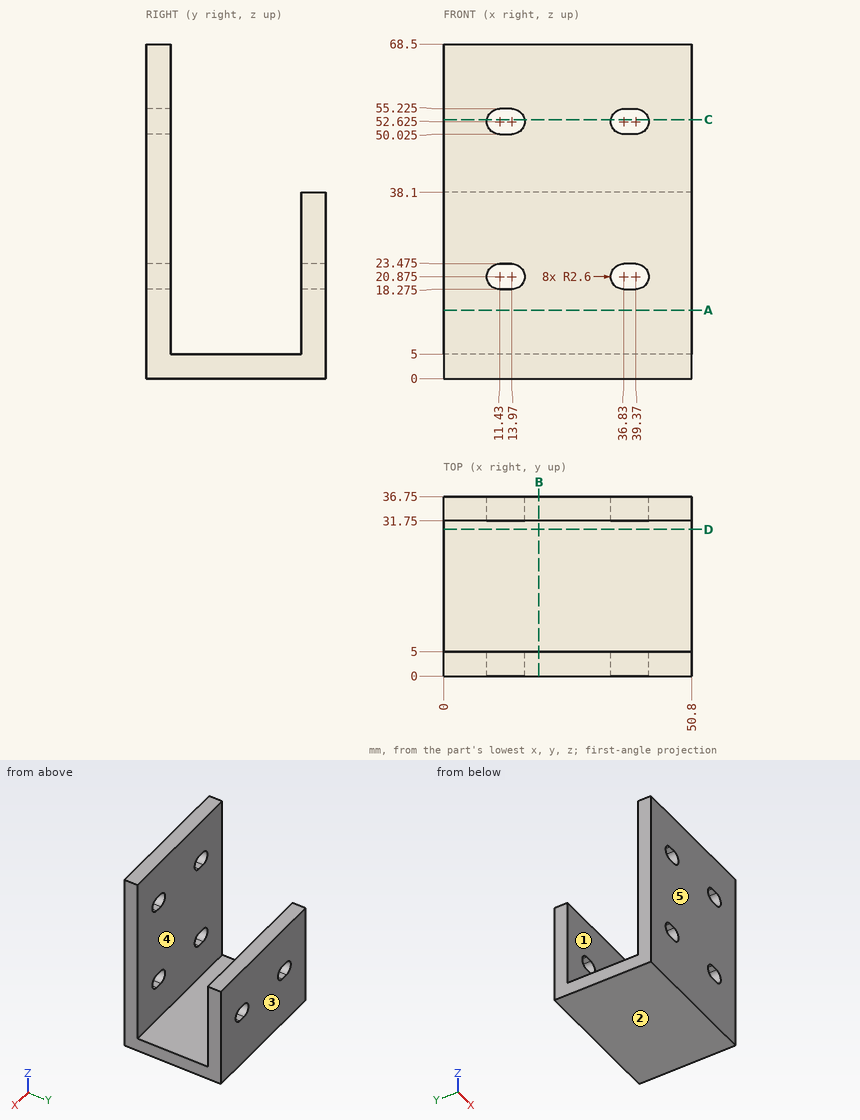
Check sheet for the drawn part. Datum: minimum x, y, z corner. Units: mm. A direction names the side the tool comes from. Round coordinates to 2 decimals unless told otherwise and drop trailing zeros. Loops run counter-clockwise (first coordinate to the right, second up) from the corner with the lowest first, then second, coordinate; pieces in that order, holes last.
Item 1: Mould release check, pull along Y, two halves, no side actions. Record for the marked faces 3, 4 and 5: pulls with the +Y half, pulls with the -Y half, needs draft (parallel to the pull), parting line crosses it, or undercut.
Item 2: Cross-section at C-C on z = 53. Record the boundary of the cut face in (x, y), then the cut area to 3 significant figures.
Item 3: Cross-section at A-A on z = 14. Record the boundary of the cut face in (x, y).
Item 4: Access from +Z, -Z, +X, -X, +Y, -Y to the whole of each face (thin tool, end or side, straight path). Record for the marked faces 1 and 2.
Item 5: Thickness scan on line 1 (Y direction, x = 6.5, z = 12.5); line 2 (Z direction, x = 40, y = 2); line 3 (Y direction, x = 10, z = 41). Record the ranges inside material, lowest first.
Item 6: Cross-section at B-B on x = 19.5. Record the boundary of the cut face in (y, z), then the cut area to 3 significant figures.
Item 7: Cross-section at D-D on y = 30. Record the boundary of the cut face in (x, z), then the cut area to 3 significant figures.
Item 8: Gauge pin test, flat ends, axial feed: pin 1 (5 mm diameter, centred on y = 28.5, z = 11.5, fed in from -X); pin 2 (2.5 mm diameter, centred on x = 27.5, y = 33.5, fed in from +Z); pin 3 (1.5 mm diameter, centred on x = 6.5, y = 21.5, fed in from +Z). Record the tip position at first contact, or that the pin passes through.
Answer sheet:
1. face 3: pulls with the +Y half
1. face 4: undercut
1. face 5: pulls with the -Y half
2. outline: (0, 0) - (8.86, 0) - (8.86, 5) - (0, 5) - close; (16.54, 0) - (34.26, 0) - (34.26, 5) - (16.54, 5) - close; (41.94, 0) - (50.8, 0) - (50.8, 5) - (41.94, 5) - close
2. area: 177 mm2
3. outline: (0, 0) - (50.8, 0) - (50.8, 5) - (0, 5) - close; (0, 31.75) - (50.8, 31.75) - (50.8, 36.75) - (0, 36.75) - close
4. face 1: +Z, +X, -X
4. face 2: -Z, +X, -X, +Y, -Y
5. line 1: y = 0 to 5, 31.75 to 36.75
5. line 2: z = 0 to 18.35, 23.4 to 50.1, 55.15 to 68.5
5. line 3: y = 0 to 5
6. outline: (0, 0) - (36.75, 0) - (36.75, 38.1) - (31.75, 38.1) - (31.75, 5) - (5, 5) - (5, 68.5) - (0, 68.5) - close
6. area: 667 mm2
7. outline: (0, 0) - (50.8, 0) - (50.8, 5) - (0, 5) - close
7. area: 254 mm2
8. pin 1: passes through
8. pin 2: stops at z = 38.1
8. pin 3: stops at z = 5
